Model file for the job. Use its own axes, mm. Face numbers are marked on the shaded views. A direction names the side the tool comes from. Give positions to 0.01 mm unless a question says otherwise; leave off trailing zeros. Loops run counter-clockwise (first coordinate to the right, second up) from the corner with the lowest first, then second, coordinate; pieces in that order, holes last. Notation, with made-up numbers: M 67,31.25 L 82,31.25 A23 ccw 82,53.25 Z; hole C 14.25,-32 d4. An arc over 180 degrees is marked long. Answer in a Markdown table with one row per item.
```python
from build123d import *

# Parameters (mm, degrees)
F1_DEPTH = 80
F3_DEPTH = 80


with BuildPart() as f1:
    # F0 (on Front) → F1 (new body)
    with BuildSketch(Plane.XZ):
        Polygon((-3.64, 10), (0, 0), (-20, 0), (-16.36, 10), (-20, 10), (-50, 10), (-50, -9.62604), (-10, -9.62604), (30, -9.62604), (30, 10), (0, 10), align=None)
    extrude(amount=-F1_DEPTH)

    # F2 (on face) → F3 (cut)
    with BuildSketch(Plane.YZ.offset(30)):
        Polygon((33.64, 10), (30, 0), (50, 0), (46.36, 10), align=None)
    extrude(amount=-F3_DEPTH, mode=Mode.SUBTRACT)


solid = f1.part
```
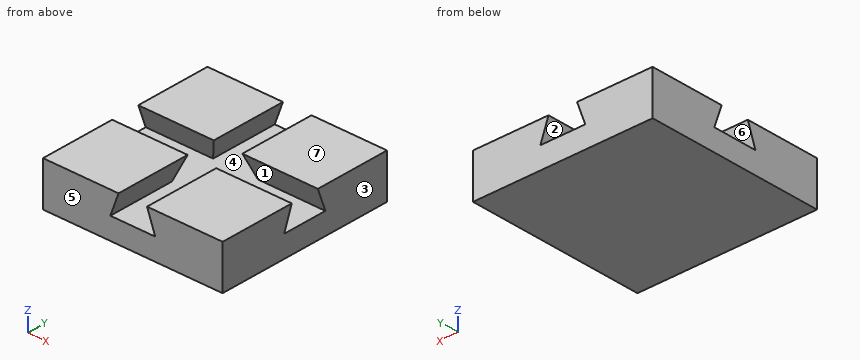
(1) Saw through at D-D, the plane y = 65. Give the cut face in (x, z).
Established:
| item | result |
|---|---|
| outline | M -50,-9.63 L 30,-9.63 L 30,10 L -3.64,10 L 0,0 L -20,0 L -16.36,10 L -50,10 Z |
(2) Saw through at C-C, the plane x = 23.5. Give the cut face in (y, z).
Established:
| item | result |
|---|---|
| outline | M 0,-9.63 L 80,-9.63 L 80,10 L 46.36,10 L 50,0 L 30,0 L 33.64,10 L 0,10 Z |
(3) Flat gauge pin, fed straight in: P1, Ø1.5, axis at x = -31, y = 37, coming from the +Z side. Where does the tip first touch, or does it go through?
Established:
| item | result |
|---|---|
| P1 | stops at z = 0 |
(4) Wall check: L1, parallel to Z at x = -37, y = 35.5; L2, parallel to X at y = 9, z = 8; L3, parallel to X at y = 54.5, z = 0.5. Give the ranges that are in metal, low to high.
Established:
| item | result |
|---|---|
| L1 | z = -9.63 to 0 |
| L2 | x = -50 to -17.09, -2.91 to 30 |
| L3 | x = -50 to -19.82, -0.18 to 30 |
(5) Mould opens along Y. For the marked faces 4, 5, 6 and 7 say: pulls with the +Y half, pulls with the -Y half, needs draft (parallel to the pull), parting line crosses it, or undercut.
Established:
| item | result |
|---|---|
| face 4 | undercut |
| face 5 | pulls with the -Y half |
| face 6 | undercut |
| face 7 | needs draft |
(6) Saw through at A-A, the plane z = 5. Give the cut face in (x, y).
Established:
| item | result |
|---|---|
| outline | M -50,0 L -18.18,0 L -18.18,31.82 L -50,31.82 Z; M -50,48.18 L -18.18,48.18 L -18.18,80 L -50,80 Z; M -1.82,0 L 30,0 L 30,31.82 L -1.82,31.82 Z; M -1.82,48.18 L 30,48.18 L 30,80 L -1.82,80 Z |
(7) Which spindle directions (+Z, -Z, +X, -X, +Y, -Y) get a long thin tool onto all of the face, cutting with end or side? Do the marked faces 1, 2 and 3. Say none if no direction does.
Established:
| item | result |
|---|---|
| face 1 | +X, -X |
| face 2 | +Y, -Y |
| face 3 | +Z, -Z, +X, +Y, -Y |
(8) Saw through at B-B, the plane y = 49. Give the cut face in (x, z).
Established:
| item | result |
|---|---|
| outline | M -50,-9.63 L 30,-9.63 L 30,0 L -50,0 Z; M -50,2.75 L -19,2.75 L -16.36,10 L -50,10 Z; M -3.64,10 L -1,2.75 L 30,2.75 L 30,10 Z |
